Geometry: final body of the model. Coordinates: model frame, mm. Coordinates: 2 decimals unless noted, no trailing zeros. Write each loop counter-clockwise with the first axis right and the second up, starting at its lowest first coordinate (ties: lowest second). Pieces come first, ordered by that corner, then holes.
Autodesk Inventor part; units mm, degrees
ref_plane "YZ Plane" through (0, 0, 0) normal (1, 0, 0) x (0, 1, 0)
ref_plane "XZ Plane" through (0, 0, 0) normal (0, 1, 0) x (-1, 0, 0)
ref_plane "XY Plane" through (0, 0, 0) normal (0, 0, 1) x (1, 0, 0)
sketch "Sketch1" plane through (0, 0, 0) normal (0, 0, 1) x (1, 0, 0)
  line L0 (-15.875, 0) -> (-12.7, 0)
  line L1 (-12.7, 0) -> (-12.7, 22.352)
  line L2 (-9.525, 25.527) -> (9.525, 25.527)
  line L3 (12.7, 22.352) -> (12.7, 0)
  line L4 (12.7, 0) -> (15.875, 0)
  line L5 (15.875, 0) -> (15.875, 25.527)
  line L6 (12.7, 28.702) -> (-12.7, 28.702)
  line L7 (-15.875, 25.527) -> (-15.875, 0)
  arc A0 (-9.525, 25.527) -> (-12.7, 22.352) centre (-9.525, 22.352) ccw
  arc A1 (12.7, 22.352) -> (9.525, 25.527) centre (9.525, 22.352) ccw
  arc A2 (-12.7, 28.702) -> (-15.875, 25.527) centre (-12.7, 25.527) ccw
  arc A3 (15.875, 25.527) -> (12.7, 28.702) centre (12.7, 25.527) ccw
  line L8 (0, 35.2315) -> (0, -5.8719)
  point P0 (0, 0)
  dimension "d0" = 28.702
  dimension "d1" = 31.75
  dimension "d2" = 3.175
  dimension "d3" = 3.175
  dimension "d4" = 3.175
extrude "Extrusion1" add sketch "Sketch1" along normal mid plane 279.4
sketch "Sketch4" plane through (15.875, 0, 139.7) normal (1, 0, 0) x (0, 0, -1)
  line L0 (139.7, -5.7404) -> (139.7, 34.4424) construction
  line L1 (-55.88, 0) -> (335.28, 0) construction
  circle A0 centre (139.7, 12.7) radius 3.175
  point P0 (139.7, 0)
  dimension "d34" = 12.7
  dimension "d35" = 0
  dimension "d36" = 6.35
extrude "Extrusion4" cut sketch "Sketch4" against normal up to surface (31.75 mm away)
pattern_linear "Rectangular Pattern3" count 15 spacing 25.4 along (0, 0, 1) count 15 spacing 25.4 along (0, 0, -1) of "Extrusion4"
equation "\"d5\" = TopLength"
equation "\"TopLength\" = 279.4"
properties part number "TopPiece" material "Aluminum 6061"
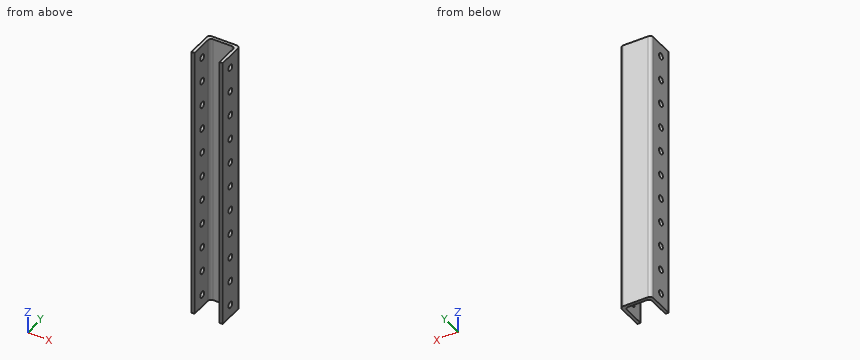
Item 1: Section D-D, the plane z = 75.5. Output: boundary loops of the cut face in (x, y) (3 decimals), plus the area to 3 significant figures.
Derived:
outline: (-15.875, 0) - (-12.7, 0) - (-12.7, 9.603) - (-15.875, 9.603) - close; (-15.875, 15.797) - (-12.7, 15.797) - (-12.7, 22.352) arc R3.175 cw to (-9.525, 25.527) - (9.525, 25.527) arc R3.175 cw to (12.7, 22.352) - (12.7, 15.797) - (15.875, 15.797) - (15.875, 25.527) arc R3.175 ccw to (12.7, 28.702) - (-12.7, 28.702) arc R3.175 ccw to (-15.875, 25.527) - close; (12.7, 0) - (15.875, 0) - (15.875, 9.603) - (12.7, 9.603) - close
area: 224 mm2
Item 2: Section C-C, the plane z = -43. Output: boundary loops of the cut face in (x, y) (3 decimals), plus the area to 3 significant figures.
Derived:
outline: (-15.875, 0) - (-12.7, 0) - (-12.7, 22.352) arc R3.175 cw to (-9.525, 25.527) - (9.525, 25.527) arc R3.175 cw to (12.7, 22.352) - (12.7, 0) - (15.875, 0) - (15.875, 25.527) arc R3.175 ccw to (12.7, 28.702) - (-12.7, 28.702) arc R3.175 ccw to (-15.875, 25.527) - close
area: 263 mm2
Item 3: Section B-B, the plane z = 127. Output: boundary loops of the cut face in (x, y) (3 decimals).
Derived:
outline: (-15.875, 0) - (-12.7, 0) - (-12.7, 9.525) - (-15.875, 9.525) - close; (-15.875, 15.875) - (-12.7, 15.875) - (-12.7, 22.352) arc R3.175 cw to (-9.525, 25.527) - (9.525, 25.527) arc R3.175 cw to (12.7, 22.352) - (12.7, 15.875) - (15.875, 15.875) - (15.875, 25.527) arc R3.175 ccw to (12.7, 28.702) - (-12.7, 28.702) arc R3.175 ccw to (-15.875, 25.527) - close; (12.7, 0) - (15.875, 0) - (15.875, 9.525) - (12.7, 9.525) - close
Item 4: Material intervals for probe 1 along X at (y, z) = (12, 66.5) (3 decimals); probe 2 along Y at (x, z) = (13.45, -101.6) (3 decimals); probe 3 along Y at (x, z) = (13.5, -70), sorted ascending.
Derived:
probe 1: x = -15.875 to -12.7, 12.7 to 15.875
probe 2: y = 0 to 9.525, 15.875 to 28.612
probe 3: y = 0 to 28.6
Item 5: Pin query (flat end, axial travel): pin 1 (4 mm diameter, centred on x = -0.5, z = -25, fed in from -Y). Return the tip coordinate at first contact, or that it passes through.
Derived:
pin 1: stops at y = 25.53
Item 6: Section A-A, the plane y = 5.5. Output: boundary loops of the cut face in (x, z) (3 decimals), plus the area to 3 significant figures.
Derived:
outline: (-15.875, -139.7) - (-12.7, -139.7) - (-12.7, 139.7) - (-15.875, 139.7) - close; (12.7, -139.7) - (15.875, -139.7) - (15.875, 139.7) - (12.7, 139.7) - close
area: 1,770 mm2
